Check sheet for the modelled part. Datum: model origin and axes. Units: mm. Face numbers are marked on the shaded views. A direction names the side the tool comes from. Give positions to 0.01 mm unless a question says otherwise; leave off trailing zeros. Loops run counter-clockwise (first coordinate to the right, second up) from the corner with the lowest first, then second, coordinate; pieces in that order, holes last. Notation, with made-up numbers: (88, 30) - (133, 30) arc R23 cw to (133, 64) - close; hole circle Ø7 at (63.25, 50). An arc over 180 degrees is marked (long way). Use one line per item in the form item = value.
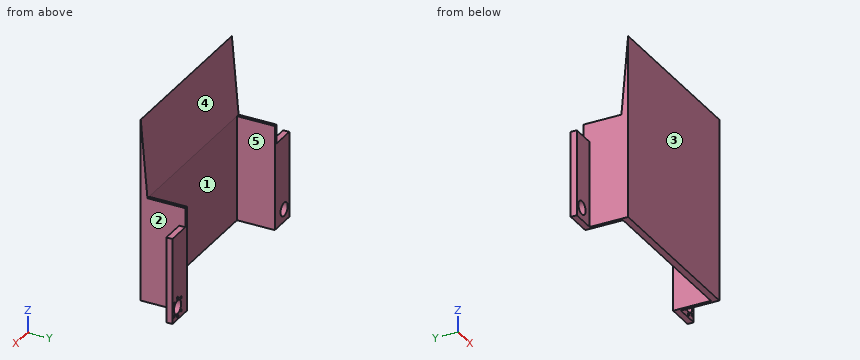
from build123d import *

# Parameters (mm, degrees)
SKETCH1_W           = 454.914
SKETCH1_H           = 381
BOSS_EXTRUDE1_DEPTH = 92.6973
SKETCH3_W           = 50.0126
SKETCH3_H           = 202.0062
CUT_EXTRUDE1_DEPTH  = 601.583496962
SKETCH4_R           = 14
CUT_EXTRUDE2_DEPTH  = 601.583496962
SKETCH5_W           = 342.1888
SKETCH5_H           = 381
CUT_EXTRUDE3_DEPTH  = 78.74
SKETCH6_W           = 178.9938
SKETCH6_H           = 79.9974
CUT_EXTRUDE4_DEPTH  = 50.0126
SKETCH7_W           = 178.9938
SKETCH7_H           = 79.9974
CUT_EXTRUDE5_DEPTH  = 50.0126
CUT_EXTRUDE6_DEPTH  = 564.647880462
SKETCH11_R          = 2.75
CUT_EXTRUDE7_DEPTH  = 601.583496962


with BuildPart() as part:
    # Sketch1 → Boss-Extrude1 (new body)
    with BuildSketch(Plane(origin=(0, 0, 0), x_dir=(1, 0, 0), z_dir=(0, 1, 0))):
        with Locations((227.457, 190.5)):
            Rectangle(SKETCH1_W, SKETCH1_H)
    extrude(amount=BOSS_EXTRUDE1_DEPTH)

    # Sketch3 → Cut-Extrude1 (cut, through all)
    with BuildSketch(Plane(origin=(0, 92.6973, 0), x_dir=(1, 0, 0), z_dir=(0, 1, 0))):
        with Locations((429.9077, 101.0031)):
            Rectangle(SKETCH3_W, SKETCH3_H)
        with Locations((25.0063, 101.0031)):
            Rectangle(SKETCH3_W, SKETCH3_H)
    extrude(amount=-CUT_EXTRUDE1_DEPTH, mode=Mode.SUBTRACT)

    # Sketch4 → Cut-Extrude2 (cut, through all)
    with BuildSketch(Plane(origin=(0, 92.6973, 0), x_dir=(1, 0, 0), z_dir=(0, 1, 0))):
        with Locations(Location((20.066, 355.092, 0), (0, 0, 270))):
            Circle(SKETCH4_R)
        with Locations(Location((434.848, 355.092, 0), (0, 0, 270))):
            Circle(SKETCH4_R)
    extrude(amount=-CUT_EXTRUDE2_DEPTH, mode=Mode.SUBTRACT)

    # Sketch5 → Cut-Extrude3 (cut)
    with BuildSketch(Plane(origin=(0, 92.6973, 0), x_dir=(1, 0, 0), z_dir=(0, 1, 0))):
        with Locations((227.457, 190.5)):
            Rectangle(SKETCH5_W, SKETCH5_H)
    extrude(amount=-CUT_EXTRUDE3_DEPTH, mode=Mode.SUBTRACT)

    # Sketch6 → Cut-Extrude4 (cut)
    with BuildSketch(Plane(origin=(454.914, 0, 0), x_dir=(0, 0, -1), z_dir=(1, 0, 0))):
        with Locations((291.5031, 39.9987)):
            Rectangle(SKETCH6_W, SKETCH6_H)
    extrude(amount=-CUT_EXTRUDE4_DEPTH, mode=Mode.SUBTRACT)

    # Sketch7 → Cut-Extrude5 (cut)
    with BuildSketch(Plane.ZY):
        with Locations((-291.5031, 39.9987)):
            Rectangle(SKETCH7_W, SKETCH7_H)
    extrude(amount=-CUT_EXTRUDE5_DEPTH, mode=Mode.SUBTRACT)

    # Sketch10 → Cut-Extrude6 (cut, through all)
    with BuildSketch(Plane(origin=(404.9014, 0, 0), x_dir=(0, 0, -1), z_dir=(1, 0, 0))):
        Polygon((0, 0), (161.899498709, 13.97), (161.899498709, 92.6973), (0, 92.6973), align=None)
    extrude(amount=-CUT_EXTRUDE6_DEPTH, mode=Mode.SUBTRACT)

    # Sketch11 → Cut-Extrude7 (cut, through all)
    with BuildSketch(Plane(origin=(0, 92.6973, 0), x_dir=(1, 0, 0), z_dir=(0, 1, 0))):
        with Locations(Location((434.848, 374.174211985, 0), (0, 0, 270))):
            Circle(SKETCH11_R)
        with Locations(Location((448.283028843, 368.609240827, 0), (0, 0, 270))):
            Circle(SKETCH11_R)
        with Locations(Location((421.412971157, 368.609240827, 0), (0, 0, 270))):
            Circle(SKETCH11_R)
        with Locations(Location((448.283028843, 341.739183142, 0), (0, 0, 270))):
            Circle(SKETCH11_R)
        with Locations(Location((434.848, 336.174211985, 0), (0, 0, 270))):
            Circle(SKETCH11_R)
        with Locations(Location((421.412971157, 341.739183142, 0), (0, 0, 270))):
            Circle(SKETCH11_R)
    extrude(amount=-CUT_EXTRUDE7_DEPTH, mode=Mode.SUBTRACT)


solid = part.part
Item 1: Gauge pin test, flat ends, axial feed: P1, Ø1.5, axis at x = 153, z = -42.5, coming from the +Y side; P2, Ø10, axis at x = 430, y = 87, coming from the +Z side; P3, Ø25, axis at x = 441.5, z = -312, coming from the -Y side. Record the tip position at first contact, or that the pin passes through.
Answer block:
P1 = 3.73
P2 = -202.01
P3 = 80
Item 2: Thickness scan on L1, parallel to X at y = 20, z = -278; L2, parallel to X at y = 5, z = -357; L3, parallel to Y at x = 180, z = -166. Record the ranges inside material, lowest first.
Answer block:
L1 = 50.01 to 56.36, 398.55 to 404.9
L2 = 50.01 to 404.9
L3 = 0 to 13.96
Item 3: Section check D-D on z = -221. Record the boundary of the cut face in (x, y).
Answer block:
outline = (0, 80) - (50.01, 80) - (50.01, 0) - (404.9, 0) - (404.9, 80) - (454.91, 80) - (454.91, 92.7) - (398.55, 92.7) - (398.55, 13.96) - (56.36, 13.96) - (56.36, 92.7) - (0, 92.7) - close
Item 4: Section check C-C on x = 410.5. Record the boundary of the cut face in (y, z).
Answer block:
outline = (80, -381) - (92.7, -381) - (92.7, -202.01) - (80, -202.01) - close
Item 5: Access from +Z, -Z, +X, -X, +Y, -Y to the whole of each face (thin tool, end or side, straight path). Record for the marked faces 4 and 5.
Answer block:
face_4 = +Z, +X, -X, +Y
face_5 = +Z, -Z, +Y
Item 6: Section check A-A on y = 59. Record the boundary of the cut face in (x, z).
Answer block:
outline = (50.01, -381) - (56.36, -381) - (56.36, -161.9) - (50.01, -161.9) - close; (398.55, -381) - (404.9, -381) - (404.9, -161.9) - (398.55, -161.9) - close
Item 7: Mould release check, pull along X, two halves, no side actions. Record for the marked faces 1, 2 and 3: released by +X, released by -X, zero draft, split by the parting line, or undercut.
Answer block:
face_1 = undercut
face_2 = released by +X
face_3 = zero draft
Item 8: Section check B-B on z = -176. Record the boundary of the cut face in (x, y), then the cut area to 3 significant figures.
Answer block:
outline = (50.01, 0) - (404.9, 0) - (404.9, 92.7) - (398.55, 92.7) - (398.55, 13.96) - (56.36, 13.96) - (56.36, 92.7) - (50.01, 92.7) - close
area = 5,950 mm2
